Model file for the job. Use its own axes, mm. Face numbers are marked on the shaded views. A direction names the side the tool comes from. Give positions to 0.01 mm unless a question says otherwise; leave off trailing zeros. Order: outer loops, then holes, each group sorted by start corner. A loop starts at its lowest first (then second) coordinate and runs counter-clockwise, first axis right, second up. Notation, with made-up numbers: (63, 59) - (102, 59) arc R15 ccw to (102, 86) - close; hole circle Ø1 at (52.5, 13). An arc over 180 degrees is marked (long way). Use CSV: the item, a comma, the result in double quotes. Start each with the question number.
(1) Band-saw the part on D-D, the plane y = -15. Give the cut face in (x, z), then the cut area to 3 significant figures.
(2) Tool access for the marked faces 1, 2 and 3: list every direction of +Z, -Z, +X, -X, +Y, -Y with a clear straight run to the whole face (end or side of a thin tool).
(3) Band-saw the part on C-C, the plane x = 13. Give the cut face in (y, z), then the cut area to 3 significant figures.
(4) Pull direction Z, two halves, no side cores. Call the marked faces 4, 5 and 6: +Z half, -Z half, draft (parallel to the pull), parting line (faces both ways), or undercut.
(5) Probe L1, parallel to Y at x = -3, z = 5.65; L2, parallel to Y at x = 10.5, z = 3.6; L3, parallel to X at y = 0.5, z = 3.55. List the from-to ranges inside material, lowest first.
(6) Drop flat-ended pins along their axis: pin 1 Ø3 at (y, z) = (-2, 4) entering from +X; pin 2 Ø1 at (x, z) = (25, 4.5) entering from +Y; pin 3 Ø1 at (x, z) = (18, 4.5) entering from -Y. Give the stop position or say it passes through.
(7) Band-saw the part on B-B, the plane y = -35. Give the cut face in (x, z).
(8) Band-saw the part on A-A, the plane z = 0.8. Give the cut face in (x, y) (3 decimals), then the cut area to 3 significant figures.
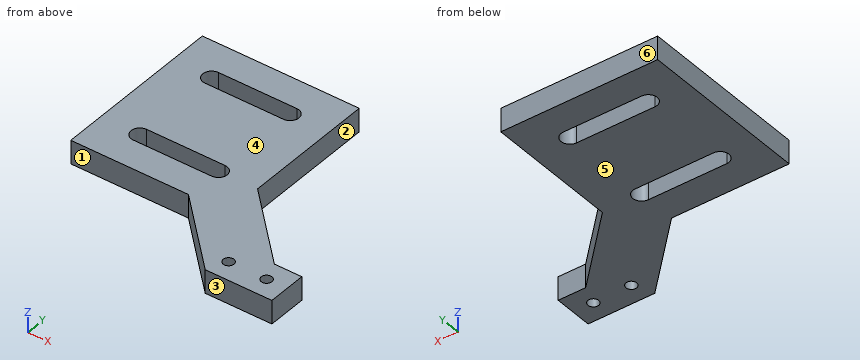
from build123d import *

# Parameters (mm, degrees)
SKETCH1_W           = 40
SKETCH1_H           = 44
BOSS_EXTRUDE1_DEPTH = 6
SKETCH3_R           = 1.375
BOSS_EXTRUDE2_DEPTH = 6


with BuildPart() as part:
    # Sketch1 → Boss-Extrude1 (new body)
    with BuildSketch(Plane.XY):
        Rectangle(SKETCH1_W, SKETCH1_H)
        with BuildLine():
            Line((-10, -9.75), (10, -9.75))
            ThreePointArc((10, -9.75), (12.25, -12), (10, -14.25))
            Line((10, -14.25), (-10, -14.25))
            ThreePointArc((-10, -14.25), (-12.25, -12), (-10, -9.75))
        make_face(mode=Mode.SUBTRACT)
        with BuildLine():
            Line((-10, 14.25), (10, 14.25))
            ThreePointArc((10, 14.25), (12.25, 12), (10, 9.75))
            Line((10, 9.75), (-10, 9.75))
            ThreePointArc((-10, 9.75), (-12.25, 12), (-10, 14.25))
        make_face(mode=Mode.SUBTRACT)
    extrude(amount=BOSS_EXTRUDE1_DEPTH)

    # Sketch3 → Boss-Extrude2 (add)
    with BuildSketch(Plane(origin=(0, 0, 0), x_dir=(-1, 0, 0), z_dir=(0, 0, -1))):
        Polygon((-20, -12), (-38, -30), (-45, -30), (-45, -40), (-28, -40), (-10, -22), (-20, -22), align=None)
        with Locations((-39.845, -35)):
            Circle(SKETCH3_R, mode=Mode.SUBTRACT)
        with Locations((-30.155, -35)):
            Circle(SKETCH3_R, mode=Mode.SUBTRACT)
    extrude(amount=-BOSS_EXTRUDE2_DEPTH)


solid = part.part
Answer block:
1,outline,"(-20, 0) - (23, 0) - (23, 6) - (-20, 6) - close"
1,area,"258 mm2"
2,face 1,"+Z, -Z, -X, -Y"
2,face 2,"+Z, -Z, +X, +Y"
2,face 3,"+Z, -Z, +X, -X, -Y"
3,outline,"(-25, 0) - (22, 0) - (22, 6) - (-25, 6) - close"
3,area,"282 mm2"
4,face 4,"+Z half"
4,face 5,"-Z half"
4,face 6,"draft"
5,L1,"y = -22 to -14.25, -9.75 to 9.75, 14.25 to 22"
5,L2,"y = -22.5 to -14.19, -9.81 to 9.81, 14.19 to 22"
5,L3,"x = -20 to 20"
6,pin 1,"stops at x = 20"
6,pin 2,"stops at y = -16.5"
6,pin 3,"stops at y = -30.5"
7,outline,"(23, 0) - (28.78, 0) - (28.78, 6) - (23, 6) - close; (31.53, 0) - (38.47, 0) - (38.47, 6) - (31.53, 6) - close; (41.22, 0) - (45, 0) - (45, 6) - (41.22, 6) - close"
8,outline,"(-20, -22) - (10, -22) - (28, -40) - (45, -40) - (45, -30) - (38, -30) - (20, -12) - (20, 22) - (-20, 22) - close; hole (-10, -14.25) - (10, -14.25) arc R2.25 ccw to (10, -9.75) - (-10, -9.75) arc R2.25 ccw to start; hole (-10, 9.75) - (10, 9.75) arc R2.25 ccw to (10, 14.25) - (-10, 14.25) arc R2.25 ccw to start; hole circle Ø2.75 at (30.155, -35); hole circle Ø2.75 at (39.845, -35)"
8,area,"1,970 mm2"
